Geometry: final body of the model. Coordinates: model frame, mm. A direction names the side the tool comes from. Give positions to 0.01 mm unless a question says otherwise; leave off trailing zeros. Write each loop counter-clockwise with the first axis right and the second up, starting at its lowest first coordinate (ties: lowest second). Pieces come first, ordered by that corner, then holes. Notation, with made-up numbers: M 54.5,53.5 L 83.5,53.5 A22 ccw 83.5,59.5 Z; hole C 62,-14.75 d2. An arc over 180 degrees is marked long. Use one line per item in the form item = value. Start each with the question number.
Item 1: Section query C-C on y = -46. Return loops of the section in (x, z), then the cut area to 3 significant figures.
Item 2: Section query B-B on x = 424. Return loops of the section in (y, z).
Item 3: Access query for faces 4 (the flat face through (399, -399, 750)), 5 (the flat face through (-401, 360, 385)), 6 (the flat face through (360, -401, 385)). Directions: +Z, -Z, +X, -X, +Y, -Y. A direction counts if a zero-diameter tool reaches every point of the face in a straight line with its end or side. Return the directions, or none.
Item 4: Material intervals for line 1 along X through (y, z) = (430.5, 479); line 2 along Z through (x, y) = (77, -463), sorted ascending. Write a range as from..to.
Item 5: Contact query for flat-ended pins moving along their axis: P1, Ø3, axis at x = 303.5, y = 50, coming from the -Z side; P2, Ø24, axis at y = -394.5, z = 419, coming from the -X side; P3, Ø24, axis at x = -382, z = 460.5, coming from the +Y side; P4, Ø3, axis at x = -23, y = -221, coming from the +Z side. Output: stop coordinate, or through.
Item 6: Section query D-D on y = -526. Return loops of the section in (x, z).
Item 7: Section query A-A on z = 515.5. Return loops of the section in (x, y), then the cut area to 3 significant figures.
Item 8: Pull-direction query (X, two-part tool) for faces 1 (the cylindrical face through (-599.967, 6.28, 14.79)), 2 (the flat face through (360, 399, 385)), 3 (the flat face through (399, -360, 385)); classes: released by +X, released by -X, zero draft, split by the parting line, or undercut.
from build123d import *

# Parameters (mm, degrees)
SKETCH_1_R      = 600
EXTRUDE_1_DEPTH = 30
SKETCH_2_W      = 80
SKETCH_2_H      = 80
EXTRUDE_2_DEPTH = 750
SKETCH_3_W      = 80
SKETCH_3_H      = 80
EXTRUDE_3_DEPTH = 750
SKETCH_4_W      = 80
SKETCH_4_H      = 80
EXTRUDE_4_DEPTH = 750
SKETCH_5_W      = 80
SKETCH_5_H      = 80
EXTRUDE_5_DEPTH = 750


with BuildPart() as part:
    # 草图1 → 凸台-拉伸1 (new body)
    with BuildSketch(Plane.XY):
        Circle(SKETCH_1_R)
    extrude(amount=EXTRUDE_1_DEPTH)

    # 草图2 → 凸台-拉伸2 (add)
    with BuildSketch(Plane.XY):
        with Locations((-400, -400)):
            Rectangle(SKETCH_2_W, SKETCH_2_H)
    extrude(amount=EXTRUDE_2_DEPTH)

    # 草图3 → 凸台-拉伸3 (add)
    with BuildSketch(Plane.XY):
        with Locations((400, -400)):
            Rectangle(SKETCH_3_W, SKETCH_3_H)
    extrude(amount=EXTRUDE_3_DEPTH)

    # 草图4 → 凸台-拉伸4 (add)
    with BuildSketch(Plane.XY):
        with Locations((-400, 400)):
            Rectangle(SKETCH_4_W, SKETCH_4_H)
    extrude(amount=EXTRUDE_4_DEPTH)

    # 草图5 → 凸台-拉伸5 (add)
    with BuildSketch(Plane.XY):
        with Locations((400, 400)):
            Rectangle(SKETCH_5_W, SKETCH_5_H)
    extrude(amount=EXTRUDE_5_DEPTH)


solid = part.part
Answer sheet:
q1.outline = M -598.23,0 L 598.23,0 L 598.23,30 L -598.23,30 Z
q1.area = 35,900 mm2
q2.outline = M -440,0 L 440,0 L 440,750 L 360,750 L 360,30 L -360,30 L -360,750 L -440,750 Z
q3.face_4 = +Z, +X, -X, +Y, -Y
q3.face_5 = +Z, +X, -X
q3.face_6 = +Z, +Y, -Y
q4.line_1 = -440..-360, 360..440
q4.line_2 = 0..30
q5.P1 = 0
q5.P2 = -440
q5.P3 = 440
q5.P4 = 30
q6.outline = M -288.66,0 L 288.66,0 L 288.66,30 L -288.66,30 Z
q7.outline = M -440,-440 L -360,-440 L -360,-360 L -440,-360 Z; M -440,360 L -360,360 L -360,440 L -440,440 Z; M 360,-440 L 440,-440 L 440,-360 L 360,-360 Z; M 360,360 L 440,360 L 440,440 L 360,440 Z
q7.area = 25,600 mm2
q8.face_1 = released by -X
q8.face_2 = undercut
q8.face_3 = zero draft
